```python
from build123d import *

# Parameters (mm, degrees)
SKETCH1_W                      = 233.3625
SKETCH1_H                      = 0.381
BASE_FLANGE1_DEPTH             = 44.45
EDGE_FLANGE1_STRIP_W           = 7.62
EDGE_FLANGE1_STRIP_H           = 0.381
EDGE_FLANGE1_STRIP_CUT_DEPTH   = 233.3625
EDGE_FLANGE1_STRIP_2_W         = 7.62
EDGE_FLANGE1_STRIP_2_H         = 0.381
EDGE_FLANGE1_STRIP_CUT_2_DEPTH = 233.3625
EDGE_FLANGE1_DEPTH             = 233.3625
EDGE_FLANGE1_BEND_DEPTH        = 233.3625
CUT_EXTRUDE1_DEPTH             = 129.834696808
FILLET1_R                      = 2.54


# Sheet-metal steps are written as plain solids
with BuildPart() as part:
    # Sketch1 → Base-Flange1 (new body)
    with BuildSketch(Plane.XY):
        with Locations((0, 0.1905)):
            Rectangle(SKETCH1_W, SKETCH1_H)
    extrude(amount=BASE_FLANGE1_DEPTH)

    # Edge-Flange1 strip (across the edge) → Edge-Flange1 strip cut (cut)
    with BuildSketch(Plane(origin=(-116.68125, 0, 0), x_dir=(0, 0, 1), z_dir=(1, 0, 0))):
        with Locations((-0.381, -0.1905)):
            Rectangle(EDGE_FLANGE1_STRIP_W, EDGE_FLANGE1_STRIP_H)
    extrude(amount=EDGE_FLANGE1_STRIP_CUT_DEPTH, mode=Mode.SUBTRACT)

    # Edge-Flange1 strip 2 (across the edge) → Edge-Flange1 strip cut 2 (cut)
    with BuildSketch(Plane(origin=(116.68125, 0, 44.45), x_dir=(0, 0, -1), z_dir=(-1, 0, 0))):
        with Locations((-0.381, -0.1905)):
            Rectangle(EDGE_FLANGE1_STRIP_2_W, EDGE_FLANGE1_STRIP_2_H)
    extrude(amount=EDGE_FLANGE1_STRIP_CUT_2_DEPTH, mode=Mode.SUBTRACT)

    # Edge-Flange1 section (across the edge) → Edge-Flange1 (add)
    with BuildSketch(Plane(origin=(-116.68125, 0, 0), x_dir=(0, 0, 1), z_dir=(1, 0, 0))):
        with BuildLine():
            Line((0, 3.048), (0, 31.369))
            Line((0, 31.369), (0.381, 31.369))
            Line((0.381, 31.369), (0.381, 3.048))
            ThreePointArc((0.381, 3.048), (1.273738531, 0.892738531), (3.429, 0))
            Line((3.429, 0), (3.429, -0.381))
            ThreePointArc((3.429, -0.381), (1.004330847, 0.623330847), (0, 3.048))
        make_face()
    extrude(amount=EDGE_FLANGE1_DEPTH)

    # Edge-Flange1 section 2 (across the edge) → Edge-Flange1 bend (add)
    with BuildSketch(Plane(origin=(116.68125, 0, 44.45), x_dir=(0, 0, -1), z_dir=(-1, 0, 0))):
        with BuildLine():
            Line((0, 3.048), (0, 31.369))
            Line((0, 31.369), (0.381, 31.369))
            Line((0.381, 31.369), (0.381, 3.048))
            ThreePointArc((0.381, 3.048), (1.273738531, 0.892738531), (3.429, 0))
            Line((3.429, 0), (3.429, -0.381))
            ThreePointArc((3.429, -0.381), (1.004330847, 0.623330847), (0, 3.048))
        make_face()
    extrude(amount=EDGE_FLANGE1_BEND_DEPTH)

    # Sketch18 → Cut-Extrude1 (cut, through all)
    with BuildSketch(Plane(origin=(0, 0.381, 0), x_dir=(1, 0, 0), z_dir=(0, 1, 0))):
        with BuildLine():
            ThreePointArc((74.530392418, -23.993293511), (88.9, -36.703), (103.269607582, -23.993293511))
            ThreePointArc((103.269607582, -23.993293511), (106.4895, -22.225), (103.269607582, -20.456706489))
            ThreePointArc((103.269607582, -20.456706489), (88.9, -7.747), (74.530392418, -20.456706489))
            ThreePointArc((74.530392418, -20.456706489), (71.3105, -22.225), (74.530392418, -23.993293511))
        make_face()
    extrude(amount=-CUT_EXTRUDE1_DEPTH, mode=Mode.SUBTRACT)

    # Fillet1
    fillet1_edges = [part.edges().sort_by_distance(p)[0] for p in [
        (-116.68125, -31.369, 0.1905),
        (116.68125, -31.369, 0.1905),
        (116.68125, -31.369, 44.2595),
        (-116.68125, -31.369, 44.2595),
    ]]
    fillet(fillet1_edges, radius=FILLET1_R)


solid = part.part
```
For this review, take the finished solid that the model builds, in its own axes (mm). A direction names the side the tool comes from. Coordinates: 2 decimals unless noted, no trailing zeros. Order: outer loops, then holes, each group sorted by start corner. A loop starts at its lowest first (then second) coordinate and runs counter-clockwise, first axis right, second up. Notation, with made-up numbers: (75.5, 18) -> (104.5, 18) arc R17 cw to (104.5, 29) -> close; hole circle Ø10 at (35, -34). An arc over 180 degrees is marked (long way). Use CSV: the item, a comma, the result in double quotes. Start each with the question number.
Item 1: Draft analysis for pull direction Z (two halves, no side actions). For faces 4 (the face through (-2, -17, 0)), 5 (the face through (2, -17, 44.069)), 6 (the face through (-2, 0.381, 22)), state which applies: pulls with the +Z half, pulls with the -Z half, needs draft (parallel to the pull), parting line crosses it, or undercut.
Item 2: We need section B-B, the plane z = 30. Give the boundary of the cut face in (x, y).
Item 3: We need section C-C, the plane x = -17. Give the boundary of the cut face in (y, z), then the cut area to 3 significant figures.
Item 4: For faces 1 (the face through (2, -17, 44.45)), 2 (the face through (89.19, 0.19, 7.75)), 3 (the face through (-2, -17, 0.381)), list the 3-axis set-ups (+Z, -Z, +X, -X, +Y, -Y) from which the entire face can be reached by the end or side of a thin tool; tool diameter is ignored.
Item 5: Wall thickness on probe 1 along Z at (x, y) = (-11, -4); probe 2 along Y at (x, z) = (-85.5, 18); probe 3 along Y at (x, z) = (-89.5, 41.5): over which ranges is each line inside the solid? List them lowest first.
Item 6: We need section A-A, the plane y = -8. Give the boundary of the cut face in (x, z).
Item 7: Insertion check: pin 1 (2 mm diameter, centred on x = -79.5, z = 32, fed in from -Y). The pin has a flat end and moves straight along its axis. Give the tip position at first contact, or say it passes through.
Derived:
1,face 4,"pulls with the -Z half"
1,face 5,"undercut"
1,face 6,"needs draft"
2,outline,"(-116.68, 0) -> (76.69, 0) -> (76.69, 0.38) -> (-116.68, 0.38) -> close; (101.11, 0) -> (116.68, 0) -> (116.68, 0.38) -> (101.11, 0.38) -> close"
3,outline,"(-31.37, 0) -> (-3.05, 0) arc R3.43 ccw to (0.38, 3.43) -> (0.38, 41.02) arc R3.43 ccw to (-3.05, 44.45) -> (-31.37, 44.45) -> (-31.37, 44.07) -> (-3.05, 44.07) arc R3.05 cw to (0, 41.02) -> (0, 3.43) arc R3.05 cw to (-3.05, 0.38) -> (-31.37, 0.38) -> close"
3,area,"39.8 mm^2"
4,face 1,"+Z, +X, -X, +Y, -Y"
4,face 2,"+Y, -Y"
4,face 3,"+X, -X, -Y"
5,probe 1,"z = 0 to 0.38, 44.07 to 44.45"
5,probe 2,"y = 0 to 0.38"
5,probe 3,"y = -0.04 to 0.35"
6,outline,"(-116.68, 0) -> (116.68, 0) -> (116.68, 0.38) -> (-116.68, 0.38) -> close; (-116.68, 44.07) -> (116.68, 44.07) -> (116.68, 44.45) -> (-116.68, 44.45) -> close"
7,pin 1,"stops at y = 0"
